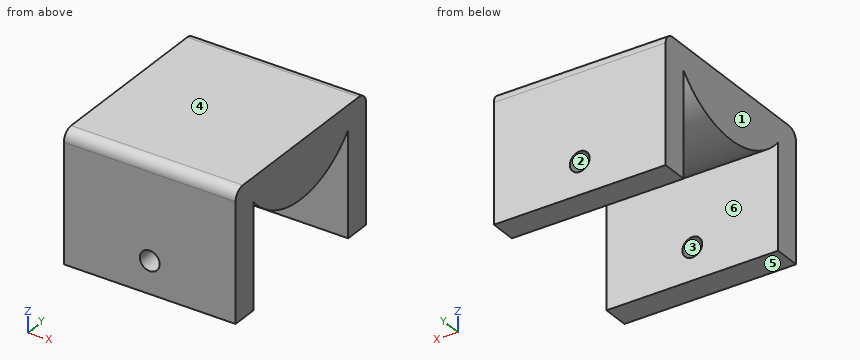
from build123d import *

# Parameters (mm, degrees)
F0_W     = 32
F0_H     = 36
F1_DEPTH = 24
F3_DEPTH = 89
F4_R     = 2
F5_R     = 2
F6_R     = 1.85
F7_DEPTH = 90


# Not quite as in the source:
# - a feature names something its author has since deleted; it is built from what else it names


with BuildPart() as f1:
    # F0 (on Top) → F1 (new body)
    with BuildSketch(Plane.XY):
        Rectangle(F0_W, F0_H)
    extrude(amount=F1_DEPTH)

    # F2 (on face) → F3 (cut)
    with BuildSketch(Plane.YZ.offset(16)):
        with BuildLine():
            ThreePointArc((13.05, 19.5), (0, 13.5), (-13.05, 19.5))
            Line((-13.05, 19.5), (-13.05, 0))
            Line((-13.05, 0), (13.05, 0))
            Line((13.05, 0), (13.05, 19.5))
        make_face()
    extrude(amount=-F3_DEPTH, mode=Mode.SUBTRACT)

    # F4
    f4_edges = [f1.edges().sort_by_distance(p)[0] for p in [
        (0, -18, 24),
    ]]
    fillet(f4_edges, radius=F4_R)

    # F5
    f5_edges = [f1.edges().sort_by_distance(p)[0] for p in [
        (0, 18, 24),
    ]]
    fillet(f5_edges, radius=F5_R)

    # F6 (on face) → F7 (cut)
    with BuildSketch(Plane.XZ.offset(18)):
        with Locations((-24, 6)):
            Circle(F6_R)
        with Locations((0, 6)):
            Circle(F6_R)
        with Locations((24, 6)):
            Circle(F6_R)
    extrude(amount=-F7_DEPTH, mode=Mode.SUBTRACT)


solid = f1.part
Design review of the part built by this model. Coordinates are the model's own, in mm. Face numbers are marked on the shaded views. A direction names the side the tool comes from. Coordinates: 2 decimals unless noted, no trailing zeros. Loops run counter-clockwise (first coordinate to the right, second up) from the corner with the lowest first, then second, coordinate; pieces in that order, holes last. Notation, with made-up numbers: (54.25, 86) -> (108.25, 86) arc R10 ccw to (108.25, 103) -> close; hole circle Ø2 at (-28.5, 31.5). An arc over 180 degrees is marked (long way). Use a Markdown table: item, result. Add a question column.
Item 1: We need section A-A, the plane z = 6. Write out the cut boundary in (x, y), and give its area (3 significant figures).
Item 2: We need section D-D, the plane x = 9.5. Write out the cut boundary in (y, z), and give its area (3 significant figures).
Item 3: The part is to be moulded in two halves that separate along X. For the marked faces 1, 2, 3 and 4, say which applies: +X half, -X half, draft (parallel to the pull), parting line (faces both ways), or undercut.
Item 4: We need section B-B, the plane x = 0. Write out the cut boundary in (y, z).
Item 5: Clearance check with flat-ended pins moving along their axes: P1, Ø6, axis at x = -6.5, y = -13, coming from the -Z side; P2, Ø12, axis at x = 11, y = 5, coming from the -Z side. State where each tip first meets the part, or that it passes through.
Item 6: Machinability: for the marked faces 5 and 6, which of the approach directions +Z, -Z, +X, -X, +Y, -Y give a long, thin tool a straight path to every point of the face, cutting with its end or side? Answer none if there is none.
Item 7: We need section C-C, the plane z = 11.25. Write out the cut boundary in (x, y).
Item 8: Wall thickness on L1, parallel to Y at x = -0.5, z = 3; L2, parallel to Z at x = 0, y = -14; L3, parallel to Y at x = 12, z = 15: over which ranges is each line inside the solid? List them lowest first. Write a range as from..to.
Numbers:
| question | item | result |
|---|---|---|
| 1 | outline | (-16, -18) -> (-1.85, -18) -> (-1.85, -13.05) -> (-16, -13.05) -> close; (-16, 13.05) -> (-1.85, 13.05) -> (-1.85, 18) -> (-16, 18) -> close; (1.85, -18) -> (16, -18) -> (16, -13.05) -> (1.85, -13.05) -> close; (1.85, 13.05) -> (16, 13.05) -> (16, 18) -> (1.85, 18) -> close |
| 1 | area | 280 mm^2 |
| 2 | outline | (-18, 0) -> (-13.05, 0) -> (-13.05, 19.5) arc R17.19 ccw to (13.05, 19.5) -> (13.05, 0) -> (18, 0) -> (18, 22) arc R2 ccw to (16, 24) -> (-16, 24) arc R2 ccw to (-18, 22) -> close |
| 2 | area | 462 mm^2 |
| 3 | face 1 | -X half |
| 3 | face 2 | undercut |
| 3 | face 3 | undercut |
| 3 | face 4 | draft |
| 4 | outline | (-18, 0) -> (-13.05, 0) -> (-13.05, 4.15) -> (-18, 4.15) -> close; (-18, 7.85) -> (-13.05, 7.85) -> (-13.05, 19.5) arc R17.19 ccw to (13.05, 19.5) -> (13.05, 7.85) -> (18, 7.85) -> (18, 22) arc R2 ccw to (16, 24) -> (-16, 24) arc R2 ccw to (-18, 22) -> close; (13.05, 0) -> (18, 0) -> (18, 4.15) -> (13.05, 4.15) -> close |
| 5 | P1 | stops at z = 0 |
| 5 | P2 | stops at z = 13.5 |
| 6 | face 5 | -Z, +X, -X, +Y, -Y |
| 6 | face 6 | -Z, +X, -X |
| 7 | outline | (-16, -18) -> (16, -18) -> (16, -13.05) -> (-16, -13.05) -> close; (-16, 13.05) -> (16, 13.05) -> (16, 18) -> (-16, 18) -> close |
| 8 | L1 | y = -18..-13.05, 13.05..18 |
| 8 | L2 | z = 0..4.15, 7.85..24 |
| 8 | L3 | y = -18..-13.05, -7.02..7.02, 13.05..18 |
